Can you work these out from the drawing? Everything is in mm from the part's minimum corner. Give positions to 0.01 mm unless a question says otherwise; leave off trailing zeros. Write each loop counter-clockwise with the first axis right and the second up, starting at its lowest first coordinate (ties: lowest second). Pieces come first, ordered by that corner, then holes. Notation, with made-up numbers: (58.5, 64) -> (75.5, 64) arc R20 cw to (75.5, 81) -> close; hole circle Ø6 at (-39.75, -6.5). An arc over 180 degrees is marked (long way). Answer as CSV lines item,"result". Start each with the question number.
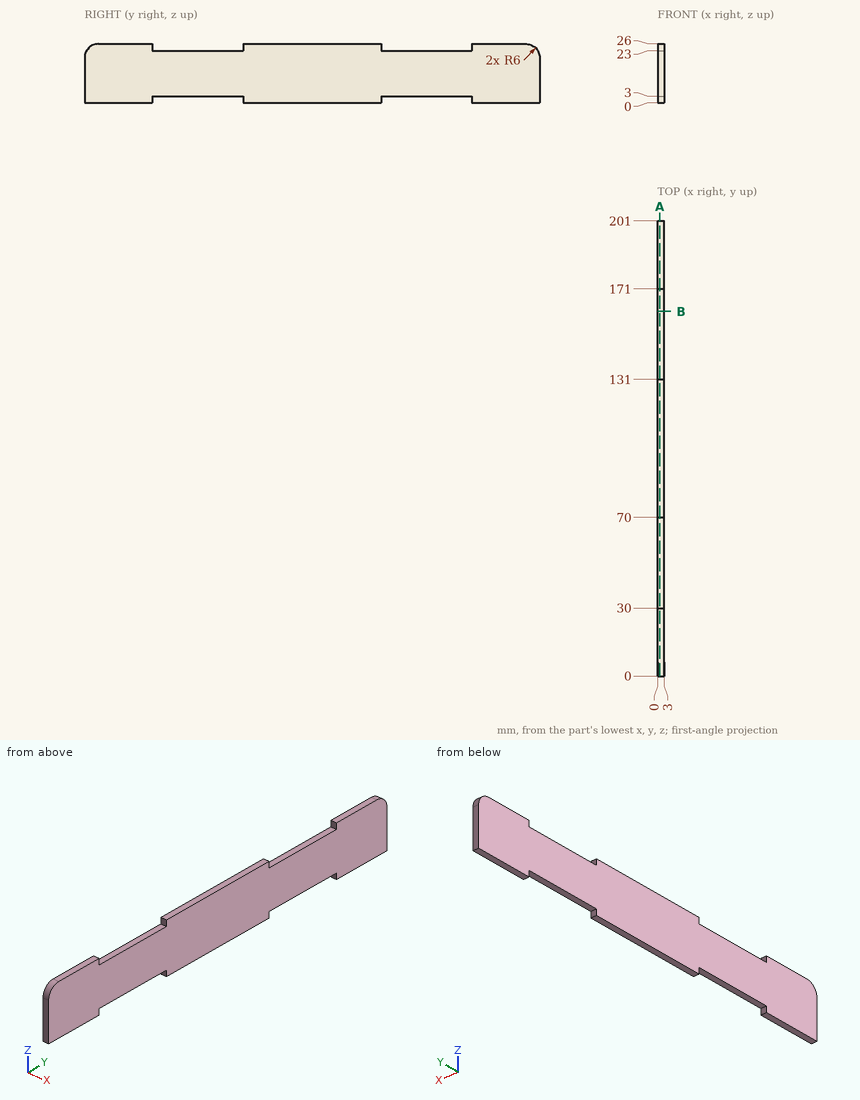
Item 1: If I drill on line 1 (Y direction, x = 1.55, z = 23.5); line 2 (Y direction, x = 1.3, z = 23.25); line 3 (Z direction, x = 1.05, y = 64.5), over which ranges is the centre line in solid material (lowest first)? Write a range as [from, to].
Item 2: I'm going to push flat-ended pins straight in: pin 1 (0.9 mm diameter, centred on x = 1, y = 59.5, fed in from -Z); pin 2 (0.9 mm diameter, centred on x = 1, y = 151.5, fed in from +Z); pin 3 (0.9 mm diameter, centred on x = 2, z = 25, fed in from +Y). Where does each tip first touch, or does it pass through?
Item 3: If we section it at B-B (y = 161): Please give me the cut outline in (x, z), and give its area (3 significant figures).
Item 4: If we section it at A-A (x = 1): Please give me the cut outline in (y, z), and give its area (3 significant figures).
Final values:
1,line 1,"[1.13, 30], [70, 131], [171, 199.87]"
1,line 2,"[0.96, 30], [70, 131], [171, 200.04]"
1,line 3,"[3, 23]"
2,pin 1,"z = 3"
2,pin 2,"z = 23"
2,pin 3,"y = 198.91"
3,outline,"(0, 3) -> (3, 3) -> (3, 23) -> (0, 23) -> close"
3,area,"60.0 mm2"
4,outline,"(0, 0) -> (30, 0) -> (30, 3) -> (70, 3) -> (70, 0) -> (131, 0) -> (131, 3) -> (171, 3) -> (171, 0) -> (201, 0) -> (201, 20) arc R6 ccw to (195, 26) -> (171, 26) -> (171, 23) -> (131, 23) -> (131, 26) -> (70, 26) -> (70, 23) -> (30, 23) -> (30, 26) -> (6, 26) arc R6 ccw to (0, 20) -> close"
4,area,"4,730 mm2"
